from build123d import *

# Parameters (mm, degrees)
CYLINDER001_R     = 2.413
CYLINDER001_DEPTH = 5.78
CYLINDER_R        = 2.4765
CYLINDER_DEPTH    = 9.67
PAD_DEPTH         = 100


with BuildPart() as cylinder001:
    # Cylinder001 → Cylinder001 (new body)
    with BuildSketch(Plane.XZ.offset(17)):
        Circle(CYLINDER001_R)
    extrude(amount=CYLINDER001_DEPTH)


with BuildPart() as cylinder:
    # Cylinder → Cylinder (new body)
    with BuildSketch(Plane.XZ.offset(3)):
        Circle(CYLINDER_R)
    extrude(amount=CYLINDER_DEPTH)


with BuildPart() as cut001:
    # Sketch → Pad (new body)
    with BuildSketch(Plane.XZ):
        with BuildLine():
            ThreePointArc((2.1082, 1.008031), (0, 2.3368), (-2.1082, 1.008031))
            Line((-2.660218, 1.008031), (-2.1082, 1.008031))
            ThreePointArc((-2.660218, 1.008031), (-2.642503, -1.053595), (-1.23687, -2.561843))
            Line((-1.016, -2.104371), (-1.23687, -2.561843))
            ThreePointArc((-1.016, -2.104371), (0, -2.3368), (1.016, -2.104371))
            Line((1.23687, -2.561843), (1.016, -2.104371))
            ThreePointArc((1.23687, -2.561843), (2.642503, -1.053595), (2.660218, 1.008031))
            Line((2.660218, 1.008031), (2.1082, 1.008031))
        make_face()
    extrude(amount=PAD_DEPTH)

    # Cut: cut Cylinder
    add(cylinder.part, mode=Mode.SUBTRACT)

    # Cut001: cut Cylinder001
    add(cylinder001.part, mode=Mode.SUBTRACT)


solid = cut001.part
CAD build for the part. Positions are in the model's coordinates, mm. A direction names the side the tool comes from. Coordinates: 2 decimals unless noted, no trailing zeros. Write each loop counter-clockwise with the first axis right and the second up, starting at its lowest first coordinate (ties: lowest second). Pieces come first, ordered by that corner, then holes. Notation, with made-up numbers: (57, -39.5) - (61, -39.5) arc R31 ccw to (61, -15.5) - close; hole circle Ø9 at (4.5, -28.75). An arc over 180 degrees is marked (long way). Use a Markdown table: item, result. Add a question column.
Item 1: Flat gauge pins, fed straight in: pin 1 (0.6 mm diameter, centred on x = 2.5, y = -55.5, fed in from +Z); pin 2 (1.5 mm diameter, centred on y = -82, z = 1, fed in from -X); pin 3 (1 mm diameter, centred on y = -69, z = -1.5, fed in from -X). Where does each tip first touch, or does it go through?
Item 2: Band-saw the part on A-A, the plane y = -15. Give the cut face in (x, z), and give its area (3 significant figures).
Item 3: Mould opens along X. For faces 1 (the face through (0.037, -14.805, 2.337)), 2 (the face through (0, -100, 0)), 3 (the face through (2.63, -49.3, -1.08)), 4 (the face through (-0.015, -60.849, -2.337)) say: pulls with the +X half, pulls with the -X half, needs draft (parallel to the pull), parting line crosses it, or undercut.
Item 4: Band-saw the part on B-B, the plane z = -0.6. Give the cut face in (x, y), and give its area (3 significant figures).
Item 5: Drill centre lines: L1, parallel to Y at x = -0.65, z = 1.4; L2, parallel to Y at x = 1.75, z = -1.7; L3, parallel to X at y = -19.5, z = -2.05. Where is each one in solid material? Low to high. Write a range as from..to.
Item 6: 3-axis set-ups, long thin cutter, end or side, ignore diameter. For faces 5 (the face through (-2.28, -19.85, -0.79)), 6 (the face through (0.037, -60.849, 2.337)): which of +Z, -Z, +X, -X, +Y, -Y reach the whole face in a straight line?
Numbers:
| question | item | result |
|---|---|---|
| 1 | pin 1 | z = 1.01 |
| 1 | pin 2 | x = -2.83 |
| 1 | pin 3 | x = -2.66 |
| 2 | outline | (-2.66, 1.01) arc R2.84 ccw to (-1.24, -2.56) - (-1.02, -2.1) arc R2.34 ccw to (1.02, -2.1) - (1.24, -2.56) arc R2.84 ccw to (2.66, 1.01) - (2.11, 1.01) arc R2.34 ccw to (-2.11, 1.01) - close |
| 2 | area | 21.2 mm2 |
| 3 | face 1 | parting line crosses it |
| 3 | face 2 | needs draft |
| 3 | face 3 | pulls with the +X half |
| 3 | face 4 | undercut |
| 4 | outline | (-2.78, -100) - (2.78, -100) - (2.78, 0) - (-2.78, 0) - close; hole (-2.4, -12.67) - (2.4, -12.67) - (2.4, -3) - (-2.4, -3) - close; hole (-2.34, -22.78) - (2.34, -22.78) - (2.34, -17) - (-2.34, -17) - close |
| 4 | area | 483 mm2 |
| 5 | L1 | -100..-22.78, -17..-12.67, -3..0 |
| 5 | L2 | -100..-12.67, -3..0 |
| 5 | L3 | -1.97..-1.27, 1.27..1.97 |
| 6 | face 5 | none |
| 6 | face 6 | +Z, +Y, -Y |
